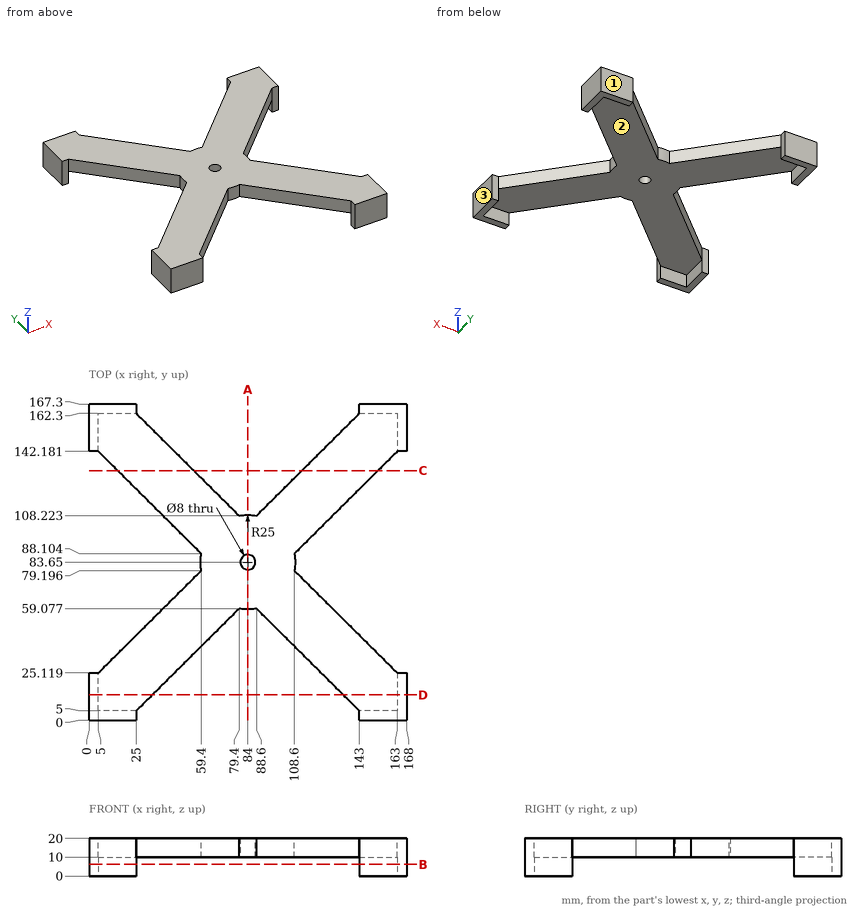
Geometry: see drawing. Coordinates: mm, zero at the bounding-box minimum. Round coordinates to 2 decimals unless told otherwise and drop trailing zeros. Loops run counter-clockwise (first coordinate to the right, second up) from the corner with the lowest first, then second, coordinate; pieces in that order, holes last. Notation, with made-up numbers: (7, -9) -> (35, -9) arc R25 ccw to (35, 19) -> close; hole circle Ø8 at (9, 31.5). An arc over 180 degrees is marked (long way). Use one line per item in the form item = value. Start each with the question number.
Item 1: Section query C-C on y = 132. Return the cut outline in (x, z).
Item 2: Material intervals for L1, parallel to Y at x = 84, z = 14; L2, parallel to Y at x = 15.5, z = 5; L3, parallel to Z at x = 60.5, y = 68, sorted ascending. Write a range as from..to.
Item 3: Mould query, pull axis X, two halves, no side actions, for the marked faces 1, 2 and 3. Classes: pulls with the +X half, pulls with the -X half, needs draft (parallel to the pull), parting line crosses it, or undercut.
Item 4: Section query D-D on y = 13.5. Return the cut outline in (x, z).
Item 5: Section query A-A on x = 84. Return the cut outline in (y, z), then the cut area to 3 significant figures.
Item 6: Section query B-B on z = 6.25. Return the cut outline in (x, y).
Item 7: Contact query for flat-ended pins moving along their axis: pin 1 Ø5 at (x, y) = (47.5, 93) entering from +Z; pin 2 Ø4 at (x, z) = (85, 8.5) entering from -Y. Output: stop coordinate, or through.
Ans:
q1.outline = (15.24, 10) -> (55.48, 10) -> (55.48, 20) -> (15.24, 20) -> close; (112.52, 10) -> (152.76, 10) -> (152.76, 20) -> (112.52, 20) -> close
q2.L1 = 58.65..79.65, 87.65..108.65
q2.L2 = 0..5, 162.3..167.3
q2.L3 = 10..20
q3.face_1 = needs draft
q3.face_2 = undercut
q3.face_3 = pulls with the +X half
q4.outline = (0, 0) -> (5, 0) -> (5, 10) -> (33.55, 10) -> (33.55, 20) -> (0, 20) -> close; (134.45, 10) -> (163, 10) -> (163, 0) -> (168, 0) -> (168, 20) -> (134.45, 20) -> close
q5.outline = (58.65, 10) -> (79.65, 10) -> (79.65, 20) -> (58.65, 20) -> close; (87.65, 10) -> (108.65, 10) -> (108.65, 20) -> (87.65, 20) -> close
q5.area = 420 mm^2
q6.outline = (0, 0) -> (25, 0) -> (25, 5) -> (5, 5) -> (5, 25.12) -> (0, 25.12) -> close; (0, 142.18) -> (5, 142.18) -> (5, 162.3) -> (25, 162.3) -> (25, 167.3) -> (0, 167.3) -> close; (143, 0) -> (168, 0) -> (168, 25.12) -> (163, 25.12) -> (163, 5) -> (143, 5) -> close; (143, 162.3) -> (163, 162.3) -> (163, 142.18) -> (168, 142.18) -> (168, 167.3) -> (143, 167.3) -> close
q7.pin_1 = through
q7.pin_2 = 58.65
